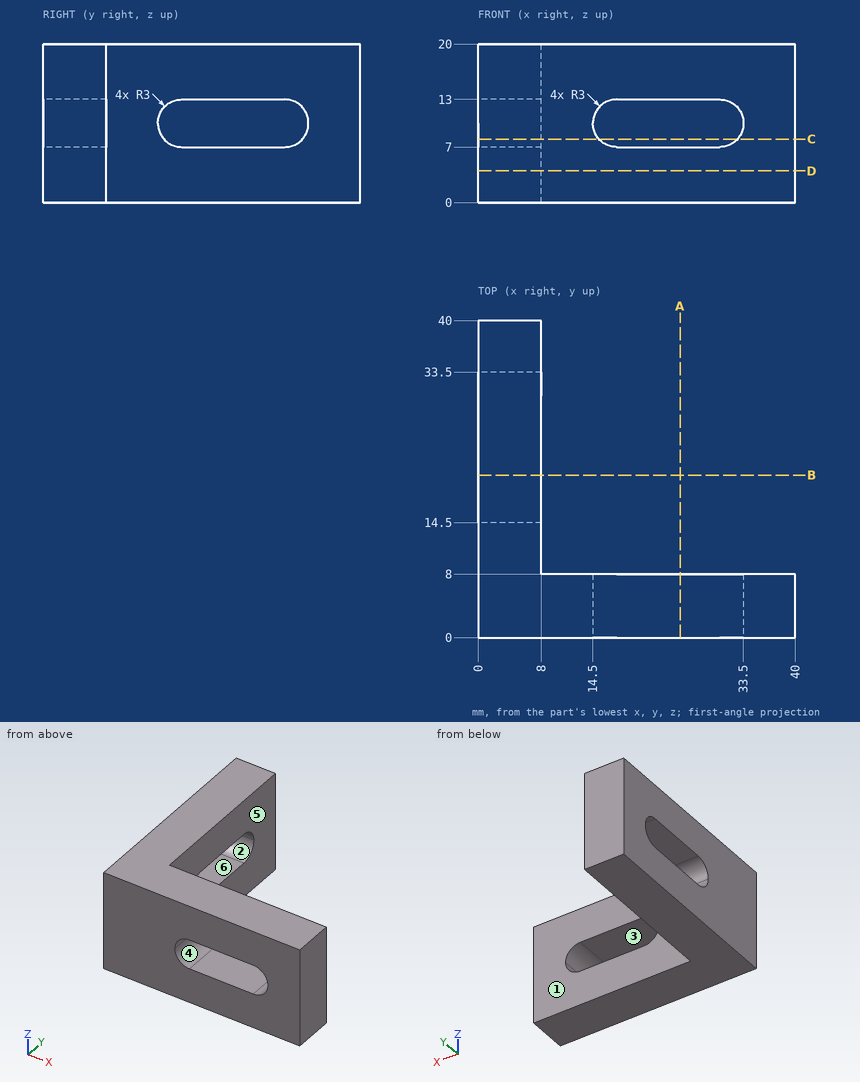
Could you check a few things on this drawing? It's one solid part, dimensions in mm from its lowest x, y, z. A direction names the side the tool comes from. Round coordinates to 2 decimals unless told otherwise and drop trailing zeros. Loops run counter-clockwise (first coordinate to the right, second up) from the corner with the lowest first, then second, coordinate; pieces in that order, holes last. Notation, with made-up numbers: M 54,9.25 L 63,9.25 A16 cw 63,30.25 Z; hole C 30.5,-2.5 d2. An arc over 180 degrees is marked long. Write each question's results on one line, items separated by ' | '. Start each with the question number.
(1) I want a section at D-D (z = 4). Please give me the cut outline in (x, y).
(2) Thinking about a two-plate mould opening in Y: for the marked faces 1, 2 and 3, which applies, pulls with the +Y half, pulls with the -Y half, needs draft (parallel to the pull), parting line crosses it, or undercut?
(3) If I drill on probe 1 along Z at (x, y) = (17.5, 3.5); probe 2 along Y at (x, z) = (34.5, 7.75), over which ranges is the centre line in solid material (lowest first)? Write a range as from..to.
(4) I want a section at A-A (x = 25.5). Please give me the cut outline in (y, z).
(5) Will these pins go through, and if not, where does the flat tip stop? P1, Ø1, axis at x = 32, z = 17, coming from the +Y side; P2, Ø8, axis at x = 11.5, y = 14.5, coming from the +Z side; P3, Ø10, axis at y = 24.5, z = 5, coming from the +X side.
(6) I want a section at C-C (z = 8). Please give me the cut outline in (x, y).
(7) On a 3-axis mill with a long thin cutter (end or side, diameter ignored), from which of +Z, -Z, +X, -X, +Y, -Y can I reach the whole of each face in a straight line? I mean the marked faces 4, 5 and 6. Say none if no direction works.
Solved:
1) outline: M 0,0 L 40,0 L 40,8 L 8,8 L 8,40 L 0,40 Z
2) face 1: pulls with the +Y half | face 2: undercut | face 3: needs draft
3) probe 1: z = 0..7, 13..20 | probe 2: y = 0..8
4) outline: M 0,0 L 8,0 L 8,7 L 0,7 Z; M 0,13 L 8,13 L 8,20 L 0,20 Z
5) P1: stops at y = 8 | P2: stops at z = 20 | P3: stops at x = 8
6) outline: M 0,0 L 15.26,0 L 15.26,8 L 8,8 L 8,15.26 L 0,15.26 Z; M 0,32.74 L 8,32.74 L 8,40 L 0,40 Z; M 32.74,0 L 40,0 L 40,8 L 32.74,8 Z
7) face 4: +Y, -Y | face 5: +Z, -Z, +X, +Y | face 6: +X, -X
